Can you work these out from the model? Positions are in its coordinate system, mm. Round coordinates to 2 decimals unless told otherwise and drop trailing zeros. Write each loop counter-clockwise with the first axis right and the second up, starting at its lowest first coordinate (ties: lowest second). Pieces come first, ordered by that corner, then holes. Notation, with made-up numbers: M 9.25,50.25 L 24.25,50.25 A28 cw 24.25,79.25 Z; hole C -11.75,-12.5 d5. An arc over 180 degrees is marked long. Answer as a JSON object with one key per item and string values. Group by question number.
1) Suppose I cut it at C-C, the plane z = 58.5. Write out the boundary of the cut face in (x, y), and give its area (3 significant figures).
2) I'm going to push a flat-ended pin straight in: pin 1 Ø1 at (y, z) = (-2.5, 51) entering from -X. Where does the tip first touch, or does it pass through?
3) Please list where these lines run through material, in increasing order: L1, parallel to Z at x = 37, y = -1.8; L2, parallel to Z at x = 38.5, y = -0.75; L3, parallel to X at y = -0.3, z = 14. Write a range as [from, to].
4) Suppose I cut it at A-A, the plane x = 12. Write out the boundary of the cut face in (y, z).
5) Suppose I cut it at D-D, the plane x = -12. Write out the boundary of the cut face in (y, z).
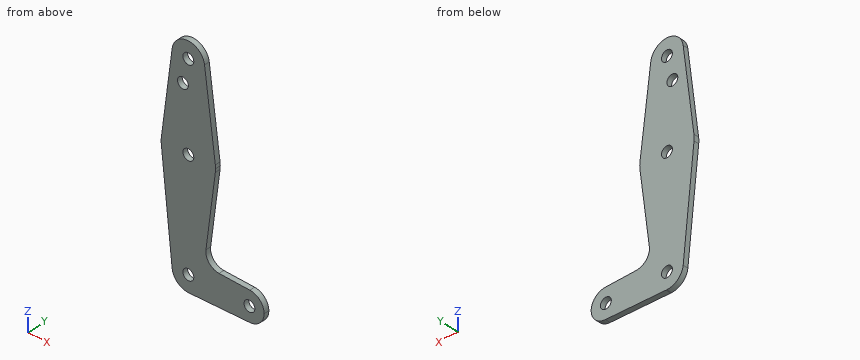
from build123d import *

# Parameters (mm, degrees)
F0_R     = 3.175
F1_DEPTH = 3.048


with BuildPart() as f1:
    # F0 (on Front) → F1 (new body)
    with BuildSketch(Plane.XZ):
        with BuildLine():
            ThreePointArc((-9.450293, 115.490625), (-0.596483, 104.793695), (9.525, 114.3))
            ThreePointArc((9.525, 114.3), (9.506305, 114.896483), (9.450293, 115.490625))
            ThreePointArc((9.450293, 115.490625), (0, 123.825), (-9.450293, 115.490625))
        make_face()
        with Locations((0, 114.3)):
            Circle(F0_R, mode=Mode.SUBTRACT)
        with BuildLine():
            ThreePointArc((9.450293, 115.490625), (9.506305, 114.896483), (9.525, 114.3))
            ThreePointArc((9.525, 114.3), (-0.596483, 104.793695), (-9.450293, 115.490625))
            Line((-9.450293, 115.490625), (-15.750488, 65.484375))
            ThreePointArc((-15.750488, 65.484375), (0, 79.375), (15.750488, 65.484375))
            Line((15.750488, 65.484375), (9.450293, 115.490625))
        make_face()
        with Locations((-3.175, 100.0252)):
            Circle(F0_R, mode=Mode.SUBTRACT)
        with BuildLine():
            ThreePointArc((15.875, 63.5), (15.843841, 64.494139), (15.750488, 65.484375))
            ThreePointArc((15.750488, 65.484375), (0, 79.375), (-15.750488, 65.484375))
            ThreePointArc((-15.750488, 65.484375), (-15.873744, 63.699705), (-15.795426, 61.9125))
            ThreePointArc((-15.795426, 61.9125), (-0.199705, 47.626256), (15.750488, 61.515625))
            ThreePointArc((15.750488, 61.515625), (15.843841, 62.505861), (15.875, 63.5))
        make_face()
        with Locations((0, 63.5)):
            Circle(F0_R, mode=Mode.SUBTRACT)
        with BuildLine():
            ThreePointArc((15.750488, 61.515625), (-0.199705, 47.626256), (-15.795426, 61.9125))
            Line((-15.795426, 61.9125), (-9.477255, -0.9525))
            ThreePointArc((-9.477255, -0.9525), (-7.063929, 6.389564), (0, 9.525))
            ThreePointArc((0, 9.525), (0.253535, 9.521625), (0.506891, 9.511503))
            ThreePointArc((0.506891, 9.511503), (6.912082, 6.553529), (9.525, 0))
            ThreePointArc((9.525, 0), (6.912082, -6.553529), (0.506891, -9.511503))
            Line((0.506891, -9.511503), (35.885598, -8.569463))
            ThreePointArc((35.885598, -8.569463), (27.084916, 0), (35.885598, 8.569463))
            Line((35.885598, 8.569463), (17.942799, 9.047231))
            ThreePointArc((17.942799, 9.047231), (12.122303, 11.815881), (10.266572, 17.988389))
            Line((10.266572, 17.988389), (15.750488, 61.515625))
        make_face()
        with BuildLine():
            ThreePointArc((0, 9.525), (-7.063929, 6.389564), (-9.477255, -0.9525))
            ThreePointArc((-9.477255, -0.9525), (-6.389564, -7.063929), (0, -9.525))
            Line((0, -9.525), (0.506891, -9.511503))
            ThreePointArc((0.506891, -9.511503), (6.912082, -6.553529), (9.525, 0))
            ThreePointArc((9.525, 0), (6.912082, 6.553529), (0.506891, 9.511503))
            Line((0.506891, 9.511503), (0, 9.525))
        make_face()
        Circle(F0_R, mode=Mode.SUBTRACT)
        with BuildLine():
            Line((0.506891, -9.511503), (0, -9.525))
            ThreePointArc((0, -9.525), (0.253535, -9.521625), (0.506891, -9.511503))
        make_face()
        with BuildLine():
            ThreePointArc((44.229916, 0), (41.799234, 5.980454), (35.885598, 8.569463))
            ThreePointArc((35.885598, 8.569463), (27.084916, 0), (35.885598, -8.569463))
            ThreePointArc((35.885598, -8.569463), (41.799234, -5.980454), (44.229916, 0))
        make_face()
        with Locations((35.657416, 0)):
            Circle(F0_R, mode=Mode.SUBTRACT)
    extrude(amount=F1_DEPTH)


solid = f1.part
Results:
{
 "1": {"outline": "M -15.45,-3.05 L 15.37,-3.05 L 15.37,0 L -15.45,0 Z", "area": "93.9 mm^2"},
 "2": {"pin 1": "x = -14.75"},
 "3": {"L1": "[-8.47, -2.88], [2.88, 8.47]", "L2": "[-8.09, -1.41], [1.41, 8.09]", "L3": "[-10.98, 10.79]"},
 "4": {"outline": "M -3.05,-9.21 L 0,-9.21 L 0,11.96 L -3.05,11.96 Z; M -3.05,31.75 L 0,31.75 L 0,95.25 L -3.05,95.25 Z"},
 "5": {"outline": "M -3.05,24.15 L 0,24.15 L 0,95.25 L -3.05,95.25 Z"}
}
